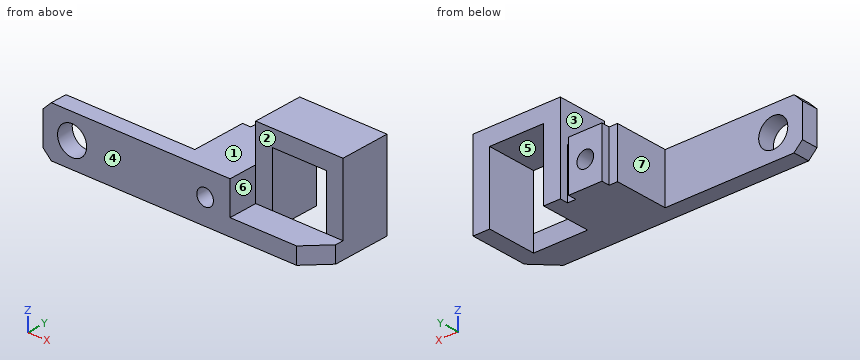
from build123d import *

# Parameters (mm, degrees)
SKETCH_1_W               = 33
SKETCH_1_H               = 12
EXTRUDE_1_DEPTH          = 4
SKETCH_1_3_W             = 12
SKETCH_1_3_H             = 12
EXTRUDE_2_DEPTH          = 19
SKETCH_2_W               = 2
SKETCH_2_H               = 12
CUT_EXTRUDE_1_DEPTH      = 2
SKETCH_3_W               = 21
SKETCH_3_H               = 21
EXTRUDE_3_DEPTH          = 19
CUT_EXTRUDE_2_DEPTH      = 58.028501646
SKETCH_5_W               = 13
SKETCH_5_H               = 13
CUT_EXTRUDE_3_DEPTH      = 56.102177815
SKETCH_6_W               = 13
SKETCH_6_H               = 4
CUT_EXTRUDE_4_DEPTH      = 12
SKETCH_7_W               = 21
SKETCH_7_H               = 7
CUT_EXTRUDE_5_DEPTH      = 17
CUT_EXTRUDE_6_DEPTH      = 54.853969213
CUT_EXTRUDE_6_DEPTH_BACK = 54.853969213
SKETCH_8_R               = 3.5
CUT_EXTRUDE_7_DEPTH      = 56.102177815
CUT_EXTRUDE_7_DEPTH_BACK = 56.102177815
SKETCH_9_R               = 2
CHAMFER_1_SIZE           = 2


with BuildPart() as part:
    # 草图1 → 凸台-拉伸1 (new body)
    with BuildSketch(Plane(origin=(0, 0, 0), x_dir=(1, 0, 0), z_dir=(0, 1, 0))):
        Rectangle(SKETCH_1_W, SKETCH_1_H)
    extrude(amount=EXTRUDE_1_DEPTH)

    # 草图1<3> → 凸台-拉伸2 (add)
    with BuildSketch(Plane(origin=(0, 0, 0), x_dir=(1, 0, 0), z_dir=(0, 1, 0))):
        with Locations((22.5, 0)):
            Rectangle(SKETCH_1_3_W, SKETCH_1_3_H)
    extrude(amount=EXTRUDE_2_DEPTH)

    # 草图2 → 切除-拉伸1 (cut)
    with BuildSketch(Plane(origin=(0, 19, 0), x_dir=(1, 0, 0), z_dir=(0, 1, 0))):
        with Locations((17.5, 0)):
            Rectangle(SKETCH_2_W, SKETCH_2_H)
        with Locations((27.5, 0)):
            Rectangle(SKETCH_2_W, SKETCH_2_H)
    extrude(amount=-CUT_EXTRUDE_1_DEPTH, mode=Mode.SUBTRACT)

    # 草图3 → 凸台-拉伸3 (add)
    with BuildSketch(Plane.XZ):
        with Locations((39, 4.5)):
            Rectangle(SKETCH_3_W, SKETCH_3_H)
    extrude(amount=-EXTRUDE_3_DEPTH)

    # 草图4 → 切除-拉伸2 (cut, through all)
    with BuildSketch(Plane.XY.offset(15)):
        Polygon((49.5, 5), (44.5, 0), (49.5, 0), align=None)
    extrude(amount=-CUT_EXTRUDE_2_DEPTH, mode=Mode.SUBTRACT)

    # 草图5 → 切除-拉伸3 (cut, through all)
    with BuildSketch(Plane(origin=(0, 19, 0), x_dir=(1, 0, 0), z_dir=(0, 1, 0))):
        with Locations((39, -4.5)):
            Rectangle(SKETCH_5_W, SKETCH_5_H)
    extrude(amount=-CUT_EXTRUDE_3_DEPTH, mode=Mode.SUBTRACT)

    # 草图6 → 切除-拉伸4 (cut)
    with BuildSketch(Plane(origin=(0, 19, 0), x_dir=(1, 0, 0), z_dir=(0, 1, 0))):
        with Locations((39, 4)):
            Rectangle(SKETCH_6_W, SKETCH_6_H)
    extrude(amount=-CUT_EXTRUDE_4_DEPTH, mode=Mode.SUBTRACT)

    # 草图7 → 切除-拉伸5 (cut)
    with BuildSketch(Plane.XY.offset(15)):
        with Locations((39, 3.5)):
            Rectangle(SKETCH_7_W, SKETCH_7_H)
    extrude(amount=-CUT_EXTRUDE_5_DEPTH, mode=Mode.SUBTRACT)

    # 草图8 → 切除-拉伸6 (cut, two sides: drawn at the far end of the back side and taken through both)
    with BuildSketch(Plane(origin=(0, 4, 0), x_dir=(1, 0, 0), z_dir=(0, 1, 0)).offset(-CUT_EXTRUDE_6_DEPTH_BACK)):
        with Locations(Location((-9.5, 0, 0), (0, 0, 270))):
            Circle(SKETCH_8_R)
    extrude(amount=CUT_EXTRUDE_6_DEPTH + CUT_EXTRUDE_6_DEPTH_BACK, mode=Mode.SUBTRACT)

    # 草图9 → 切除-拉伸7 (cut, two sides: drawn at the far end of the back side and taken through both)
    with BuildSketch(Plane(origin=(0, 19, 0), x_dir=(1, 0, 0), z_dir=(0, 1, 0)).offset(-CUT_EXTRUDE_7_DEPTH_BACK)):
        with Locations(Location((22.5, 0, 0), (0, 0, 270))):
            Circle(SKETCH_9_R)
    extrude(amount=CUT_EXTRUDE_7_DEPTH + CUT_EXTRUDE_7_DEPTH_BACK, mode=Mode.SUBTRACT)

    # 倒角1
    chamfer_1_edges = [part.edges().sort_by_distance(p)[0] for p in [
        (-16.5, 2, 6),
        (-16.5, 2, -6),
    ]]
    chamfer(chamfer_1_edges, length=CHAMFER_1_SIZE)


solid = part.part
Geometry: final body of the model. Coordinates: model frame, mm. Face numbers are marked on the shaded views. A direction names the side the tool comes from. Coordinates: 2 decimals unless noted, no trailing zeros. Order: outer loops, then holes, each group sorted by start corner. A loop starts at its lowest first (then second) coordinate and runs counter-clockwise, first axis right, second up.
1) Section D-D (z = 0). Return loops of the section in (x, y).
Result sheet:
outline: (-16.5, 0) - (-13, 0) - (-13, 4) - (-16.5, 4) - close; (-6, 0) - (20.5, 0) - (20.5, 19) - (18.5, 19) - (18.5, 17) - (16.5, 17) - (16.5, 4) - (-6, 4) - close; (24.5, 0) - (28.5, 0) - (28.5, 7) - (32.5, 7) - (32.5, 19) - (28.5, 19) - (28.5, 17) - (26.5, 17) - (26.5, 19) - (24.5, 19) - close; (45.5, 7) - (49.5, 7) - (49.5, 19) - (45.5, 19) - close
2) Draft query along X for the marked faces 4, 5, 6 and 7. Return one class per face: released by +X, released by -X, zero draft, split by the parting line, or undercut.
Result sheet:
face 4: zero draft
face 5: undercut
face 6: released by +X
face 7: released by -X
3) Section B-B (z = 9.75). Return loops of the section in (x, y).
Result sheet:
outline: (28.5, 7) - (32.5, 7) - (32.5, 19) - (28.5, 19) - close; (45.5, 7) - (49.5, 7) - (49.5, 19) - (45.5, 19) - close
4) Section A-A (x = 22.5). Return loops of the section in (y, z), then the cut area to 3 significant figures.
Result sheet:
outline: (0, -6) - (19, -6) - (19, -2) - (0, -2) - close; (0, 2) - (19, 2) - (19, 6) - (0, 6) - close
area: 152 mm2
5) Section C-C (y = 3.25). Return loops of the section in (x, z), then the cut area to 3 significant figures.
Result sheet:
outline: (-16.5, -4) - (-14.5, -6) - (47.75, -6) - (47.75, -2) - (28.5, -2) - (28.5, 6) - (-14.5, 6) - (-16.5, 4) - close; hole circle Ø7 at (-9.5, 0); hole circle Ø4 at (22.5, 0)
area: 562 mm2
6) Set-up query: the marked faces 1, 2 and 3. Return all of +Z, -Z, +X, -X, +Y, -Y with unobstructed straight access to the full face (end or side cutting, diameter ignored); none if empty.
Result sheet:
face 1: +Z, -X, +Y, -Y
face 2: +Z, +X, -Y
face 3: +Z, +Y
7) First-contact query: P1, Ø6, axis at x = -7, z = -0.5, coming from the +Y side; P2, Ø5.5, axis at x = 34, y = 3, coming from the +Z side; P3, Ø7.5, axis at y = 2.5, z = 3, coming from the +X side. Flat tips, straight axial feed; report the tip coordinate or a pass-through.
Result sheet:
P1: stops at y = 4
P2: stops at z = -2
P3: stops at x = 28.5
8) Ray query, probe 1 along X at (y, z) = (2.55, 0); probe 2 along Z at (x, y) = (-9.5, 2); probe 3 along Z at (x, y) = (22.5, 4). Return the intervals inside material, ascending.
Result sheet:
probe 1: x = -16.5 to -13, -6 to 20.5, 24.5 to 28.5
probe 2: z = -6 to -3.5, 3.5 to 6
probe 3: z = -6 to -2, 2 to 6
